```python
from build123d import *

# Parameters (mm, degrees)
ESBO_O1_W             = 33
ESBO_O1_H             = 12
CORTE_EXTRUS_O2_DEPTH = 49.187135213
CORTE_EXTRUS_O3_DEPTH = 49.187135213
PADR_OCIRCULAR2_COUNT = 20


with BuildPart() as part:
    # Esboço1 → Revolução1 (revolve)
    with BuildSketch(Plane(origin=(0, 0, 0), x_dir=(1, 0, 0), z_dir=(0, 1, 0)), mode=Mode.PRIVATE) as revolu_o1_sk:
        with Locations((16.5, 6)):
            Rectangle(ESBO_O1_W, ESBO_O1_H)
    revolve(revolu_o1_sk.sketch.rotate(Axis((0, 0, 0), (0, 0, 1)), 180), axis=Axis((0, 0, 0), (0, 0, 1)))

    # Esboço3 → Corte-extrusão2 (cut, through all)
    with BuildSketch(Plane(origin=(0, 0, -12), x_dir=(-1, 0, 0), z_dir=(0, 0, -1))):
        with BuildLine():
            Line((-2.236067977, 2), (2.236067977, 2))
            ThreePointArc((2.236067977, 2), (0, -3), (-2.236067977, 2))
        make_face()
    extrude(amount=-CORTE_EXTRUS_O2_DEPTH, mode=Mode.SUBTRACT)

    # Esboço2 → Corte-extrusão3 (cut, through all)
    with BuildSketch(Plane.XY):
        with BuildLine():
            ThreePointArc((1.489278925, 26.206717637), (0, 26.249), (-1.489278925, 26.206717637))
            ThreePointArc((-1.489278925, 26.206717637), (-2.448651415, 29.690511169), (-4.401620335, 32.730762038))
            ThreePointArc((-4.401620335, 32.730762038), (0, 33.0254), (4.401620335, 32.730762038))
            ThreePointArc((4.401620335, 32.730762038), (2.448651415, 29.690511169), (1.489278925, 26.206717637))
        make_face()
    corte_extrus_o3 = extrude(amount=-CORTE_EXTRUS_O3_DEPTH, mode=Mode.SUBTRACT)

    # PadrãoCircular2: Corte-extrusão3 ×20 about axis
    padr_ocircular2_axis = Axis((0, 0, 0), (0, 0, 1))
    for i in range(1, PADR_OCIRCULAR2_COUNT):
        add(corte_extrus_o3.rotate(padr_ocircular2_axis, i * 360 / PADR_OCIRCULAR2_COUNT), mode=Mode.SUBTRACT)


solid = part.part
```
The listing builds one solid part. Answer for the finished solid, in the listing's coordinates (mm). A direction names the side the tool comes from. Give positions to 0.01 mm unless a question says otherwise; leave off trailing zeros. Write each loop counter-clockwise with the first axis right and the second up, starting at its lowest first coordinate (ties: lowest second). Pieces come first, ordered by that corner, then holes. Notation, with made-up numbers: (60, 16) - (113, 16) arc R23 cw to (113, 33) - close; hole circle Ø7 at (15.25, -8.5). An arc over 180 degrees is marked (long way). Use one line per item in the form item = value. Start each with the question number.
1) Find section D-D on y = -18. Determine the outline of the cut face in (x, z), plus the area to 3 significant figures.
2) Find section C-C on x = 27. Determine the outline of the cut face in (y, z), plus the area to 3 significant figures.
3) A tool of negligible diameter and unlimited length cuts with its end or side. For faces 1 (the face through (25.494, 15.478, -5.916)), 2 (the face through (-2.42, 29.63, -5.92)), 3 (the face through (22.55, 19.38, -5.92)), 4 (the face through (-29.72, 2.46, -5.92)), 5 (the face through (-2.46, -29.72, -5.92)), from which of +Z, -Z, +X, -X, +Y, -Y can it reach the whole face along a straight path? Write none if from no direction.
4) The mould has two halves that part along X. Classify faces 6 (the face through (25.395, -15.457, -5.916)), 7 (the face through (29.63, 2.42, -5.92)), 8 (the face through (-27.43, -11.46, -5.92)): pulls with the +X half, pulls with the -X half, needs draft (parallel to the pull), parting line crosses it, or undercut.
5) Consider line 1 along Y through (x, z) = (0, -2.75); line 2 along Y through (x, z) = (-28, -3.5); line 3 along Y through (x, z) = (-28.5, -7.25). Determine where each line is inside the solid, lowest interval first. Write a range as from..to.
6) Flat-ended cylindrical pins translate along their axes: pin 1 Ø6 at (y, z) = (23.5, -9) entering from -X; pin 2 Ø6 at (y, z) = (17.5, -2.5) entering from -X. Find the tip coordinate at first contact, or state that the pin passes through.
7) Find section B-B on y = 0. Determine the outline of the cut face in (x, z).
8) Find section A-A on x = 0. Determine the outline of the cut face in (y, z), plus the area to 3 significant figures.
Geometry results:
q1.outline = (-21.61, -12) - (21.61, -12) - (21.61, 0) - (-21.61, 0) - close
q1.area = 519 mm2
q2.outline = (-15.69, -12) - (-11.09, -12) - (-11.09, 0) - (-15.69, 0) - close; (-6.89, -12) - (-1.61, -12) - (-1.61, 0) - (-6.89, 0) - close; (1.61, -12) - (6.89, -12) - (6.89, 0) - (1.61, 0) - close; (11.09, -12) - (15.69, -12) - (15.69, 0) - (11.09, 0) - close
q2.area = 237 mm2
q3.face_1 = +Z, -Z
q3.face_2 = +Z, -Z, +Y
q3.face_3 = +Z, -Z, +X
q3.face_4 = +Z, -Z, -X
q3.face_5 = +Z, -Z, -Y
q4.face_6 = undercut
q4.face_7 = pulls with the +X half
q4.face_8 = pulls with the -X half
q5.line_1 = -26.25..-3, 2..26.25
q5.line_2 = -15.73..-12, -6.91..-1.84, 1.84..6.91, 12..15.73
q5.line_3 = -15.72..-12.54, -6.89..-1.99, 1.99..6.89, 12.54..15.72
q6.pin_1 = -23.89
q6.pin_2 = -29.64
q7.outline = (-26.25, -12) - (-3, -12) - (-3, 0) - (-26.25, 0) - close; (3, -12) - (26.25, -12) - (26.25, 0) - (3, 0) - close
q8.outline = (-26.25, -12) - (-3, -12) - (-3, 0) - (-26.25, 0) - close; (2, -12) - (26.25, -12) - (26.25, 0) - (2, 0) - close
q8.area = 570 mm2
